```python
from build123d import *

# Parameters (mm, degrees)
SKETCH1_R           = 30
SKETCH1_R_2         = 22.5
BOSS_EXTRUDE1_DEPTH = 20
SKETCH2_W           = 50
SKETCH2_H           = 20
BOSS_EXTRUDE2_DEPTH = 7.5
SKETCH4_W           = 14.39860727
SKETCH4_H           = 10
CUT_EXTRUDE1_DEPTH  = 20
CUT_EXTRUDE3_DEPTH  = 5
SKETCH8_R           = 3
CUT_EXTRUDE4_DEPTH  = 10
BOSS_EXTRUDE3_DEPTH = 7.5
CUT_EXTRUDE5_DEPTH  = 5


with BuildPart() as part:
    # Sketch1 → Boss-Extrude1 (new body)
    with BuildSketch(Plane(origin=(0, 0, 0), x_dir=(1, 0, 0), z_dir=(0, 1, 0))):
        with Locations(Location((0, 0, 0), (0, 0, 270))):
            Circle(SKETCH1_R)
        with Locations(Location((0, 0, 0), (0, 0, 270))):
            Circle(SKETCH1_R_2, mode=Mode.SUBTRACT)
    extrude(amount=BOSS_EXTRUDE1_DEPTH)

    # Sketch2 → Boss-Extrude2 (add)
    with BuildSketch(Plane(origin=(22.5, 0, 0), x_dir=(0, 0, -1), z_dir=(1, 0, 0))):
        with Locations((0, 10)):
            Rectangle(SKETCH2_W, SKETCH2_H)
    extrude(amount=BOSS_EXTRUDE2_DEPTH)

    # Sketch4 → Cut-Extrude1 (cut)
    with BuildSketch(Plane(origin=(0, 0, 0), x_dir=(1, 0, 0), z_dir=(0, 1, 0))):
        with Locations((-26.790895642, 0)):
            Rectangle(SKETCH4_W, SKETCH4_H)
    extrude(amount=CUT_EXTRUDE1_DEPTH, mode=Mode.SUBTRACT)

    # Sketch7 → Cut-Extrude3 (cut)
    with BuildSketch(Plane(origin=(30, 0, 0), x_dir=(0, 0, -1), z_dir=(1, 0, 0))):
        Polygon((-1, 9.625), (-20, 2.5), (20, 2.5), (1, 9.625), (1, 10.375), (20, 17.5), (-20, 17.5), (-1, 10.375), align=None)
    extrude(amount=-CUT_EXTRUDE3_DEPTH, mode=Mode.SUBTRACT)

    # Sketch8 → Cut-Extrude4 (cut)
    with BuildSketch(Plane(origin=(30, 0, 0), x_dir=(0, 0, -1), z_dir=(1, 0, 0))):
        with Locations((0, 10)):
            Circle(SKETCH8_R)
    extrude(amount=-CUT_EXTRUDE4_DEPTH, mode=Mode.SUBTRACT)

    # Sketch9 → Boss-Extrude3 (add)
    with BuildSketch(Plane(origin=(30, 0, 0), x_dir=(0, 0, -1), z_dir=(1, 0, 0))):
        Polygon((-25, 20), (0, 34.357764991), (25, 20), align=None)
    extrude(amount=-BOSS_EXTRUDE3_DEPTH)

    # Sketch10 → Cut-Extrude5 (cut)
    with BuildSketch(Plane(origin=(30, 0, 0), x_dir=(0, 0, -1), z_dir=(1, 0, 0))):
        Polygon((-20, 20.088403301), (20, 20.088403301), (0, 29.990964176), align=None)
    extrude(amount=-CUT_EXTRUDE5_DEPTH, mode=Mode.SUBTRACT)


solid = part.part
```
Can you work these out from the model? Positions are in its coordinate system, mm. A direction names the side the tool comes from. Give positions to 0.01 mm unless a question says otherwise; leave off trailing zeros. Order: outer loops, then holes, each group sorted by start corner. A loop starts at its lowest first (then second) coordinate and runs counter-clockwise, first axis right, second up. Notation, with made-up numbers: (-36.5, 71.25) - (17.5, 71.25) arc R11 cw to (17.5, 87.25) - close; hole circle Ø6 at (-14, -1). An arc over 180 degrees is marked (long way). Use a Markdown table: item, result. Add a question column.
Q1. Please list where these lines run through material, in increasing order: line 1 along Y through (x, z) = (26.5, 0); line 2 along Z through (x, y) = (0, 11.75); line 3 along Z through (x, y) = (24, 10).
Q2. On a 3-axis mill with a long thin cutter (end or side, diameter ignored), from which of +Z, -Z, +X, -X, +Y, -Y can I reach the whole of each face in a straight line? I mean faces 1 (the flat face through (26, 10, -25)), 2 (the flat face through (-4, 20, -23)), 3 (the flat face through (27.54, 25.11, 9.86)). Say none if no direction works.
Q3. If we section it at D-D on x = 18: Write out the boundary of the cut face in (y, z).
Q4. If we mould it in two halves opening along Y, with no side actions, what happens to faces 4 (the flat face through (26, 10, 25)), 5 (the flat face through (28, 2.5, 0)), 6 (the flat face through (-4, 20, 23))? For each: released by +Y, released by -Y, zero draft, split by the parting line, or undercut.
Q5. I'm going to push flat-ended pins straight in: pin 1 (1 mm diameter, centred on y = 26, z = 11.5, fed in from -X); pin 2 (9 mm diameter, centred on x = -9.5, z = 16.5, fed in from +Y); pin 3 (4 mm diameter, centred on x = -25, y = 11.5, fed in from +Z); pin 4 (5.5 mm diameter, centred on y = 10, z = 0, fed in from -X). Where does each tip first touch, or does it pass through?
Q6. If we section it at C-C on y = 10: Write out the boundary of the cut face in (x, z), plus the area to 3 significant figures.
Q7. If we section it at B-B on z = 14.5: Write out the boundary of the cut face in (x, y).
Q8. If we section it at A-A on x = 0: Write out the boundary of the cut face in (y, z).
Answers follow:
| question | item | result |
|---|---|---|
| 1 | line 1 | y = 0 to 2.5, 17.5 to 20.09, 29.99 to 34.36 |
| 1 | line 2 | z = -30 to -22.5, 22.5 to 30 |
| 1 | line 3 | z = -25 to -3, 3 to 25 |
| 2 | face 1 | -Z, +X, +Y, -Y |
| 2 | face 2 | +Z, -Z, -X, +Y |
| 2 | face 3 | +X |
| 3 | outline | (0, -24) - (20, -24) - (20, -13.5) - (0, -13.5) - close; (0, 13.5) - (20, 13.5) - (20, 24) - (0, 24) - close |
| 4 | face 4 | zero draft |
| 4 | face 5 | undercut |
| 4 | face 6 | released by +Y |
| 5 | pin 1 | stops at x = 22.5 |
| 5 | pin 2 | stops at y = 20 |
| 5 | pin 3 | stops at z = 19.26 |
| 5 | pin 4 | passes through |
| 6 | outline | (-29.58, -5) arc R30 ccw to (22.5, -19.84) - (22.5, -25) - (30, -25) - (30, -3) - (22.3, -3) arc R22.5 cw to (-21.94, -5) - close; (-29.58, 5) - (-21.94, 5) arc R22.5 cw to (22.3, 3) - (30, 3) - (30, 25) - (22.5, 25) - (22.5, 19.84) arc R30 ccw to start |
| 6 | area | 1,290 mm^2 |
| 7 | outline | (-26.26, 0) - (-17.2, 0) - (-17.2, 20) - (-26.26, 20) - close; (17.2, 0) - (30, 0) - (30, 2.5) - (25, 2.5) - (25, 4.56) - (30, 4.56) - (30, 15.44) - (25, 15.44) - (25, 17.5) - (30, 17.5) - (30, 20.09) - (25, 20.09) - (25, 22.81) - (30, 22.81) - (30, 26.03) - (22.5, 26.03) - (22.5, 20) - (17.2, 20) - close |
| 8 | outline | (0, -30) - (20, -30) - (20, -22.5) - (0, -22.5) - close; (0, 22.5) - (20, 22.5) - (20, 30) - (0, 30) - close |
